from build123d import *

# Parameters (mm, degrees)
SKETCH1_R           = 75
SKETCH1_R_2         = 55
BOSS_EXTRUDE1_DEPTH = 21.45
SKETCH3_R           = 2.8
CUT_EXTRUDE1_DEPTH  = 27.8


with BuildPart() as part:
    # Sketch1 → Boss-Extrude1 (new body)
    with BuildSketch(Plane.XY):
        Circle(SKETCH1_R)
        Circle(SKETCH1_R_2, mode=Mode.SUBTRACT)
    extrude(amount=BOSS_EXTRUDE1_DEPTH)

    # Sketch3 → Cut-Extrude1 (cut)
    with BuildSketch(Plane(origin=(0, 0, 0), x_dir=(-1, 0, 0), z_dir=(0, 0, -1))):
        with Locations((0, 65)):
            Circle(SKETCH3_R)
        with Locations((56.291651246, -32.5)):
            Circle(SKETCH3_R)
        with Locations((-56.291651246, -32.5)):
            Circle(SKETCH3_R)
    extrude(amount=-CUT_EXTRUDE1_DEPTH, mode=Mode.SUBTRACT)


solid = part.part
Part model, mm, in its own coordinate system. Give positions to 0.01 mm unless a question says otherwise; leave off trailing zeros. Loops run counter-clockwise (first coordinate to the right, second up) from the corner with the lowest first, then second, coordinate; pieces in that order, holes last.
(1) Drill centre lines: line 1 along Y through (x, z) = (0, 17.25); line 2 along Y through (x, z) = (-22, 10); line 3 along Y through (x, z) = (45, 7.5). Where is each one in solid material? Low to high.
Return value:
line 1: y = -75 to -55, 55 to 62.2, 67.8 to 75
line 2: y = -71.7 to -50.41, 50.41 to 71.7
line 3: y = -60 to -31.62, 31.62 to 60
(2) Pull direction X, two halves, no side cores. Call faces 1 (the cylindrical face through (-11.923, -53.692, 10.575)), 2 (the flat face through (-22.57, 50.35, 0)), 3 (the cylindrical face through (-9.764, 74.362, 10.575)): pulls with the +X half, pulls with the -X half, needs draft (parallel to the pull), parting line crosses it, or undercut.
Return value:
face 1: undercut
face 2: needs draft
face 3: parting line crosses it
(3) Pin check, flat tips, straight feed: pin 1 (12 mm diameter, centred on x = 54.5, z = 3.5, fed in from -Y); pin 2 (1 mm diameter, centred on y = -20.5, z = 18.5, fed in from -X); pin 3 (10 mm diameter, centred on y = -53, z = 17, fed in from +X). Stop position of each tip, or through.
Return value:
pin 1: stops at y = -57.21
pin 2: stops at x = -72.28
pin 3: stops at x = 57.63
(4) Band-saw the part on B-B (x = 0). Write the cut outline in (y, z).
Return value:
outline: (-75, 0) - (-55, 0) - (-55, 21.45) - (-75, 21.45) - close; (55, 0) - (62.2, 0) - (62.2, 21.45) - (55, 21.45) - close; (67.8, 0) - (75, 0) - (75, 21.45) - (67.8, 21.45) - close
(5) Band-saw the part on D-D (x = 20). Write the cut outline in (y, z).
Return value:
outline: (-72.28, 0) - (-51.23, 0) - (-51.23, 21.45) - (-72.28, 21.45) - close; (51.23, 0) - (72.28, 0) - (72.28, 21.45) - (51.23, 21.45) - close
(6) Band-saw the part on C-C (z = 10.25). Write the cut outline in (x, y).
Return value:
outline: circle Ø150 at (0, 0); hole circle Ø5.6 at (-56.29, -32.5); hole circle Ø110 at (0, 0); hole circle Ø5.6 at (0, 65); hole circle Ø5.6 at (56.29, -32.5)
(7) Band-saw the part on A-A (y = 0). Write the cut outline in (x, z).
Return value:
outline: (-75, 0) - (-55, 0) - (-55, 21.45) - (-75, 21.45) - close; (55, 0) - (75, 0) - (75, 21.45) - (55, 21.45) - close
